from build123d import *

# Parameters (mm, degrees)
SKETCH1_W           = 12
SKETCH1_H           = 12
BOSS_EXTRUDE1_DEPTH = 3
SKETCH2_W           = 4
SKETCH2_H           = 4
BOSS_EXTRUDE2_DEPTH = 4
SKETCH3_R           = 1
CUT_EXTRUDE1_DEPTH  = 3
FILLET2_R           = 0.5
SKETCH4_W           = 0.2
SKETCH4_H           = 1
BOSS_EXTRUDE3_DEPTH = 4
CHAMFER1_SIZE       = 1


with BuildPart() as part:
    # Sketch1 → Boss-Extrude1 (new body)
    with BuildSketch(Plane(origin=(0, 0, 0), x_dir=(1, 0, 0), z_dir=(0, 1, 0))):
        Rectangle(SKETCH1_W, SKETCH1_H)
    extrude(amount=BOSS_EXTRUDE1_DEPTH)

    # Sketch2 → Boss-Extrude2 (add)
    with BuildSketch(Plane(origin=(0, 3, 0), x_dir=(1, 0, 0), z_dir=(0, 1, 0))):
        Rectangle(SKETCH2_W, SKETCH2_H)
    extrude(amount=BOSS_EXTRUDE2_DEPTH)

    # Sketch3 → Cut-Extrude1 (cut)
    with BuildSketch(Plane(origin=(0, 7, 0), x_dir=(1, 0, 0), z_dir=(0, 1, 0))):
        Circle(SKETCH3_R)
    extrude(amount=-CUT_EXTRUDE1_DEPTH, mode=Mode.SUBTRACT)

    # Fillet2
    fillet2_edges = [part.edges().sort_by_distance(p)[0] for p in [
        (2, 5, 2),
        (2, 5, -2),
        (-2, 5, -2),
        (-2, 5, 2),
    ]]
    fillet(fillet2_edges, radius=FILLET2_R)

    # Sketch4 → Boss-Extrude3 (add)
    with BuildSketch(Plane.XZ):
        with Locations((-5.9, -2.5)):
            Rectangle(SKETCH4_W, SKETCH4_H)
        with Locations((-5.9, 2.5)):
            Rectangle(SKETCH4_W, SKETCH4_H)
        with Locations((5.9, 2.5)):
            Rectangle(SKETCH4_W, SKETCH4_H)
        with Locations((5.9, -2.5)):
            Rectangle(SKETCH4_W, SKETCH4_H)
    extrude(amount=BOSS_EXTRUDE3_DEPTH)

    # Chamfer1
    chamfer1_edges = [part.edges().sort_by_distance(p)[0] for p in [
        (6, 1.5, 6),
        (-6, 1.5, 6),
        (-6, 1.5, -6),
        (6, 1.5, -6),
    ]]
    chamfer(chamfer1_edges, length=CHAMFER1_SIZE)


solid = part.part
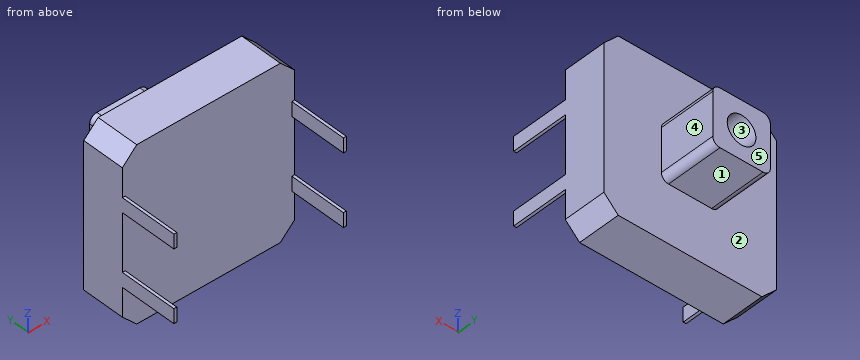
The model under review builds one solid part; all positions refer to its coordinate system, in mm. Face numbers are marked on the shaded views. A direction names the side the tool comes from. Coordinates: 2 decimals unless noted, no trailing zeros. Write each loop counter-clockwise with the first axis right and the second up, starting at its lowest first coordinate (ties: lowest second). Pieces come first, ordered by that corner, then holes. Notation, with made-up numbers: (-19, -21) - (3, -21) arc R11 ccw to (3, -11) - close; hole circle Ø8 at (-10.75, 54.5). An arc over 180 degrees is marked (long way). Answer as a JSON object with one key per item and string values. Group by question number.
1. To check wall thickness, follow probe 1 along Z at (x, y) = (0, 4.8); probe 2 along X at (y, z) = (-2.75, -2.5). State the ranges of each line that lie inside material, in increasing order.
2. Mouldability with a two-part tool opening along Z and no side actions: class the marked faces 1, 2 and 3 as pulls with the +Z half, pulls with the -Z half, needs draft (parallel to the pull), parting line crosses it, or undercut.
3. Add section B-B (y = -1). Give the boundary of the cut face in (x, z), plus the area to 3 significant figures.
4. Machinability: for the marked faces 4 and 5, which of the approach directions +Z, -Z, +X, -X, +Y, -Y give a long, thin tool a straight path to every point of the face, cutting with its end or side? Answer none if there is none.
5. Add section C-C (x = 0). Give the boundary of the cut face in (y, z), plus the area to 3 significant figures.
6. Add section A-A (z = -2.5). Give the boundary of the cut face in (x, y).
7. Clearance check with flat-ended pins moving along their axes: pin 1 Ø2.5 at (x, y) = (0.5, 5.5) entering from -Z; pin 2 Ø0.9 at (y, z) = (4.5, 0.5) entering from +X; pin 3 Ø3 at (x, z) = (-1.5, 0) entering from -Y. State where each tip first meets the part, or that it passes through.
8. Add section D-D (y = 5.5). Give the boundary of the cut face in (x, z).
Findings:
{
 "1": {"probe 1": "-2 to -1, 1 to 2", "probe 2": "-6 to -5.8, 5.8 to 6"},
 "2": {"face 1": "pulls with the -Z half", "face 2": "needs draft", "face 3": "undercut"},
 "3": {"outline": "(-6, -3) - (-5.8, -3) - (-5.8, -2) - (-6, -2) - close; (-6, 2) - (-5.8, 2) - (-5.8, 3) - (-6, 3) - close; (5.8, -3) - (6, -3) - (6, -2) - (5.8, -2) - close; (5.8, 2) - (6, 2) - (6, 3) - (5.8, 3) - close", "area": "0.800 mm²"},
 "4": {"face 4": "+Z, -Z, +X, +Y", "face 5": "+Z, -Z, +X, -X, +Y"},
 "5": {"outline": "(0, -6) - (3, -6) - (3, -2) - (7, -2) - (7, -1) - (4, -1) - (4, 1) - (7, 1) - (7, 2) - (3, 2) - (3, 6) - (0, 6) - close", "area": "46.0 mm²"},
 "6": {"outline": "(-6, -4) - (-5.8, -4) - (-5.8, 0) - (5.8, 0) - (5.8, -4) - (6, -4) - (6, 3) - (-6, 3) - close"},
 "7": {"pin 1": "z = -2", "pin 2": "x = 2", "pin 3": "y = 0"},
 "8": {"outline": "(-2, -1.5) arc R0.5 ccw to (-1.5, -2) - (1.5, -2) arc R0.5 ccw to (2, -1.5) - (2, 1.5) arc R0.5 ccw to (1.5, 2) - (-1.5, 2) arc R0.5 ccw to (-2, 1.5) - close; hole circle Ø2 at (0, 0)"}
}
